```python
from build123d import *

# Parameters (mm, degrees)
BOSS_EXTRUDE1_DEPTH      = 3
SKETCH2_R                = 4
SKETCH2_R_2              = 1.6
CUT_EXTRUDE1_DEPTH       = 13
SKETCH3_W                = 26
SKETCH3_H                = 3
BOSS_EXTRUDE2_DEPTH      = 29
CUT_EXTRUDE3_START       = -20
CUT_EXTRUDE3_OUTLINE_R   = 1.6
CUT_EXTRUDE3_OUTLINE_R_2 = 5
CUT_EXTRUDE3_DEPTH       = 3


# Read off the part's stored shape, not the designer's step: Cut-Extrude3
with BuildPart() as part:
    # Sketch1 → Boss-Extrude1 (new body)
    with BuildSketch(Plane.XY):
        with BuildLine():
            Line((0, 0), (0, -20))
            Line((0, -20), (26, -20))
            Line((26, -20), (26, 0))
            ThreePointArc((26, 0), (13, 13), (0, 0))
        make_face()
    extrude(amount=BOSS_EXTRUDE1_DEPTH)

    # Sketch2 → Cut-Extrude1 (cut)
    with BuildSketch(Plane.XY.offset(3)):
        with Locations((13, 0)):
            Circle(SKETCH2_R)
        with Locations((4.5, 0)):
            Circle(SKETCH2_R_2)
        with Locations((21.5, 0)):
            Circle(SKETCH2_R_2)
    extrude(amount=-CUT_EXTRUDE1_DEPTH, mode=Mode.SUBTRACT)

    # Sketch3 → Boss-Extrude2 (add)
    with BuildSketch(Plane(origin=(0, 0, 0), x_dir=(-1, 0, 0), z_dir=(0, 0, -1))):
        with Locations((-13, -18.5)):
            Rectangle(SKETCH3_W, SKETCH3_H)
    extrude(amount=BOSS_EXTRUDE2_DEPTH)

    # Cut-Extrude3 outline → Cut-Extrude3 (cut)
    with BuildSketch(Plane(origin=(0, 0, 0), x_dir=(1, 0, 0), z_dir=(0, 1, 0)).offset(CUT_EXTRUDE3_START)):
        with Locations((5, 20)):
            Circle(CUT_EXTRUDE3_OUTLINE_R)
        with Locations((21, 6)):
            Circle(CUT_EXTRUDE3_OUTLINE_R)
        with Locations((21, 20)):
            Circle(CUT_EXTRUDE3_OUTLINE_R)
        with Locations((13, 13)):
            Circle(CUT_EXTRUDE3_OUTLINE_R_2)
        with Locations((5, 6)):
            Circle(CUT_EXTRUDE3_OUTLINE_R)
    extrude(amount=CUT_EXTRUDE3_DEPTH, mode=Mode.SUBTRACT)


solid = part.part
```
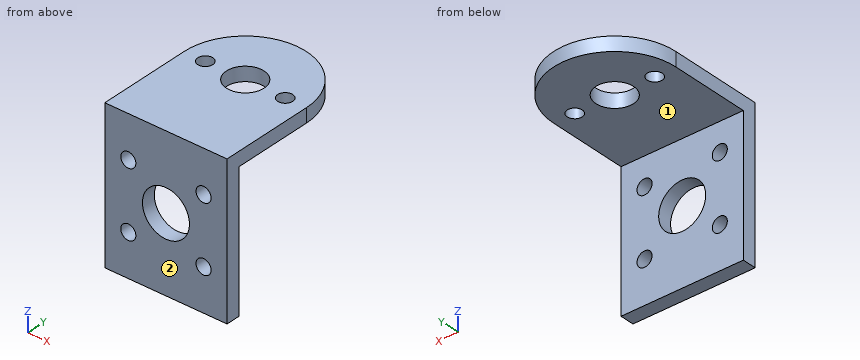
Verification items for the finished model (mm, model axes). Face numbers are marked on the shaded views. A direction names the side the tool comes from. Round coordinates to 2 decimals unless told otherwise and drop trailing zeros. Write each loop counter-clockwise with the first axis right and the second up, starting at its lowest first coordinate (ties: lowest second). Pieces come first, ordered by that corner, then holes. Notation, with made-up numbers: (1.5, 33.25) -> (58.5, 33.25) arc R20 cw to (58.5, 42.25) -> close; hole circle Ø5 at (26, -10). An arc over 180 degrees is marked (long way). Write each question's results on one line, items separated by ' | '. Start each with the question number.
1. Cross-section at A-A (z = -13). Enter the section's corners in (x, y), then the cut area to 3 significant figures.
2. Cross-section at B-B (z = -6). Enter the section's corners in (x, y).
3. Depth check by flat-ended pin: P1, Ø1.5, axis at x = 12.5, y = 8.5, coming from the -Z side; P2, Ø3.5, axis at x = 21.5, y = 0, coming from the +Z side; P3, Ø3, axis at x = 7.5, z = -23, coming from the +Y side. Enter the tip coordinate at first touch or a pass-through.
4. Cross-section at C-C (x = 13). Enter the section's corners in (y, z).
5. Set-up check for the marked faces 1 and 2: record each of +Z, -Z, +X, -X, +Y, -Y from which the full face is reachable in a straight line by a thin tool's end or side.
6. Material ranges on probe 1 along Z at (x, y) = (21, -18.05); probe 2 along X at (y, z) = (-17.9, -20); probe 3 along Z at (x, y) = (20.75, 6.5), recorded low to high. Write a range as from..to.
7. Cross-section at D-D (x = 21). Enter the section's corners in (y, z), then the cut area to 3 significant figures.
Solutions:
1) outline: (0, -20) -> (8, -20) -> (8, -17) -> (0, -17) -> close; (18, -20) -> (26, -20) -> (26, -17) -> (18, -17) -> close | area: 48.0 mm2
2) outline: (0, -20) -> (3.4, -20) -> (3.4, -17) -> (0, -17) -> close; (6.6, -20) -> (19.4, -20) -> (19.4, -17) -> (6.6, -17) -> close; (22.6, -20) -> (26, -20) -> (26, -17) -> (22.6, -17) -> close
3) P1: stops at z = 0 | P2: stops at z = 3 | P3: stops at y = -17
4) outline: (-20, -29) -> (-17, -29) -> (-17, -18) -> (-20, -18) -> close; (-20, -8) -> (-17, -8) -> (-17, 0) -> (-4, 0) -> (-4, 3) -> (-20, 3) -> close; (4, 0) -> (13, 0) -> (13, 3) -> (4, 3) -> close
5) face 1: -Z, +X, -X, +Y | face 2: +Z, -Z, +X, -X, -Y
6) probe 1: z = -29..-21.6, -18.4..-7.6, -4.4..3 | probe 2: x = 0..3.4, 6.6..19.4, 22.6..26 | probe 3: z = 0..3
7) outline: (-20, -29) -> (-17, -29) -> (-17, -21.6) -> (-20, -21.6) -> close; (-20, -18.4) -> (-17, -18.4) -> (-17, -7.6) -> (-20, -7.6) -> close; (-20, -4.4) -> (-17, -4.4) -> (-17, 0) -> (-1.52, 0) -> (-1.52, 3) -> (-20, 3) -> close; (1.52, 0) -> (10.25, 0) -> (10.25, 3) -> (1.52, 3) -> close | area: 149 mm2
